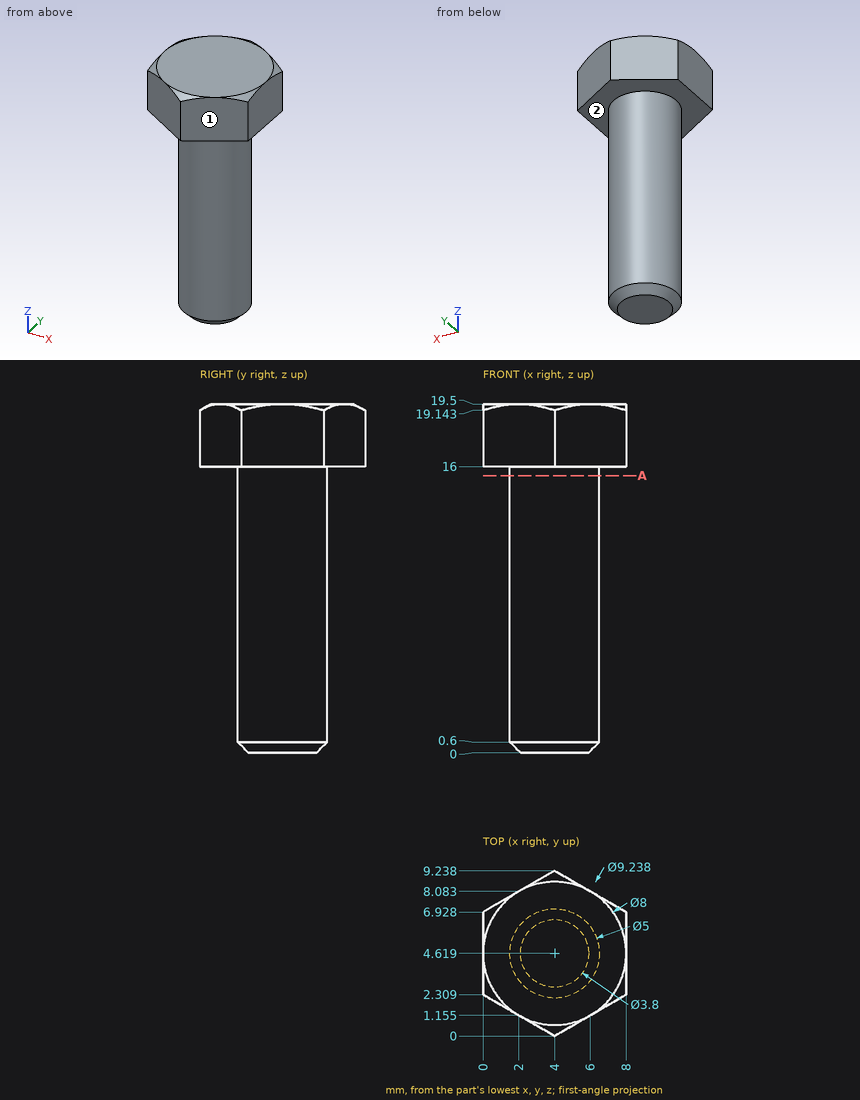
The drawing under review shows one solid part. Ordinate dimensions are in mm from its lowest x, y, z. A direction names the side the tool comes from. Give positions to 0.01 mm unless a question says otherwise; leave off trailing zeros. Write each loop counter-clockwise with the first axis right and the second up, starting at its lowest first coordinate (ties: lowest second). Pieces come first, ordered by that corner, then holes. Notation, with made-up numbers: (77.5, 37.25) - (113.5, 37.25) arc R20 ccw to (113.5, 45.25) - close; hole circle Ø4 at (59.5, -7). An arc over 180 degrees is marked (long way). Answer in a Markdown table with one row per item. Add a question column.
1. Tool access review of the marked faces 1 and 2: name each direction out of +Z, -Z, +X, -X, +Y, -Y from which nothing blocks a thin tool from reaching the whole face with its end or side.
2. Insertion check: P1, Ø1.5, axis at x = 5.5, z = 11.5, coming from the -Y side; P2, Ø1, axis at y = 5.5, z = 7.5, coming from the +X side; P3, Ø3, axis at x = 5.5, z = 4, coming from the +Y side. Each pin has a flat end and moves straight along its axis. Give the tip position at first contact, or say it passes through.
3. We need section A-A on z = 15.5. Write out the cut boundary in (x, y).
4. Wall thickness on line 1 along Z through (x, y) = (7, 7.25); line 2 along X through (y, z) = (3, 9.75) (1 decimal); line 3 along Y through (x, z) = (4.5, 18.25): over which ranges is each line inside the solid? List them lowest first. Write a range as [from, to].
Ans:
| question | item | result |
|---|---|---|
| 1 | face 1 | +Z, -Z, +X, -Y |
| 1 | face 2 | -Z |
| 2 | P1 | stops at y = 2.23 |
| 2 | P2 | stops at x = 6.47 |
| 2 | P3 | stops at y = 7.12 |
| 3 | outline | circle Ø5 at (4, 4.62) |
| 4 | line 1 | z = [16, 19.5] |
| 4 | line 2 | x = [2.1, 5.9] |
| 4 | line 3 | y = [0.29, 8.95] |
